from build123d import *

# Parameters (mm, degrees)
F0_R      = 15
F1_DEPTH  = 150
F2_R      = 14
F3_DEPTH  = 150
F4_W      = 14
F4_H      = 20
F9_W      = 7
F9_H      = 30
F10_DEPTH = 250


with BuildPart() as f1:
    # F0 (on Top) → F1 (new body)
    with BuildSketch(Plane.XY):
        Circle(F0_R)
    extrude(amount=F1_DEPTH)

    # F2 (on face) → F3 (cut, through all)
    with BuildSketch(Plane.XY.offset(150)):
        Circle(F2_R)
    extrude(amount=-F3_DEPTH, mode=Mode.SUBTRACT)

    # F6: sweep along a path in F5
    with BuildLine(Plane.YZ) as f6_path:
        Line((0, 35.6896594167), (-15, 35.6896594167))
        Line((-15, 35.6896594167), (-226.3578921556, 152.8566330671))
    # F4 (on Front) → F6 (sweep)
    with BuildSketch(Plane.XZ):
        with Locations((0, 25)):
            Rectangle(F4_W, F4_H)
    sweep(path=f6_path.line, transition=Transition.RIGHT)


with BuildPart() as f10:
    # F9 (on face) → F10 (new body)
    with BuildSketch(Plane(origin=(0, 0, 0), x_dir=(-1, 0, 0), z_dir=(0, 0.8660254038, 0.5))):
        with Locations((3.5, 36.4281994849)):
            Rectangle(F9_W, F9_H)
        with Locations((-3.5, 36.4281994849)):
            Rectangle(F9_W, F9_H)
    extrude(amount=F10_DEPTH)

    # F11: cut F1
    add(f1.part, mode=Mode.SUBTRACT)


solid = f1.part
The listing builds one solid part. Answer for the finished solid, in the listing's coordinates (mm). A direction names the side the tool comes from. Give positions to 0.01 mm unless a question says otherwise; leave off trailing zeros. Write each loop counter-clockwise with the first axis right and the second up, starting at its lowest first coordinate (ties: lowest second). Pieces come first, ordered by that corner, then holes.
1) Section D-D (y = -56) is taken. Write down the section's boundary in (x, z).
2) For a pull along X with two mould halves and no side action, classify faces 1 (the face through (0, -7, 35)), 2 (the face through (7, -117, 83)), 3 (the face through (0.098, -231.473, 143.63)) as pulls with the +X half, pulls with the -X half, needs draft (parallel to the pull), parting line crosses it, or undercut.
3) Section B-B (z = 83.5) is taken. Write down the section's boundary in (x, y), and give its area (3 significant figures).
4) Section C-C (z = 23.5) is taken. Write down the section's boundary in (x, y), and give its area (3 significant figures).
5) Section A-A (x = 0) is taken. Write down the section's boundary in (y, z).
6) Find the intervals of material crossed by L1, parallel to Y at x = 0, z = 49; L2, parallel to Y at x = 0, z = 101.5; L3, parallel to Y at x = -10.25, z = 67, in increasing order.
7) Given P1, Ø9.5, axis at y = -8, z = 22, coming from the -X side; P2, Ø5, axis at x = -3.5, y = -198.5, coming from the +Z side; P3, Ø3.5, axis at y = -4, z = 25, coming from the +X side, each flat-ended and moving along its own axis, determine where each tip first touches the part or whether it passes through.
8) A tool of negligible diameter and unlimited length cuts with its end or side. For faces 4 (the face through (0.1, -122.42, 94.45)), 5 (the face through (0, -7, 15)), 6 (the face through (-7, -6, 25)), from which of +Z, -Z, +X, -X, +Y, -Y can it reach the whole face along a straight path? Write none if from no direction.
Response:
1. outline: (-7, 34.76) - (7, 34.76) - (7, 57.63) - (-7, 57.63) - close
2. face 1: undercut
2. face 2: pulls with the +X half
2. face 3: needs draft
3. outline: circle Ø30 at (0, 0); (-7, -143.92) - (7, -143.92) - (7, -102.67) - (-7, -102.67) - close; hole circle Ø28 at (0, 0)
3. area: 669 mm2
4. outline: (-7, -35.68) - (7, -35.68) - (7, -13.27) arc R15 ccw (long way) to (-7, -13.27) - close; hole (-7, -12.12) - (-7, 0) - (7, 0) - (7, -12.12) arc R14 ccw (long way) to start
4. area: 576 mm2
5. outline: (-236.39, 134.76) - (-20.35, 15) - (-15, 15) - (-15, 0) - (-14, 0) - (-14, 15) - (0, 15) - (0, 35) - (-14, 35) - (-14, 150) - (-15, 150) - (-15, 35) - (-15.18, 35) - (-226.69, 152.25) - close; (14, 0) - (15, 0) - (15, 150) - (14, 150) - close
6. L1: y = -81.68 to -40.43, -15 to -14, 14 to 15
6. L2: y = -176.39 to -135.14, -15 to -14, 14 to 15
6. L3: y = -10.95 to -9.54, 9.54 to 10.95
7. P1: stops at x = -14.64
7. P2: stops at z = 138.01
7. P3: stops at x = 14.83
8. face 4: +Z, +X, -X
8. face 5: -Z
8. face 6: +Z, -Z
